from build123d import *

# Parameters (mm, degrees)
SKETCH_1_R               = 11
SKETCH_1_R_2             = 1.25
EXTRUDE_1_DEPTH          = 2
SKETCH_2_R               = 5
SKETCH_2_R_2             = 2.5
EXTRUDE_2_DEPTH          = 10
CUT_EXTRUDE_1_REACH      = 21.647
CUT_EXTRUDE_1_END_RADIUS = 5
SKETCH_3_R               = 1.5


with BuildPart() as part:
    # 草圖1 → 填料-伸長1 (new body)
    with BuildSketch(Plane(origin=(0, 0, 0), x_dir=(1, 0, 0), z_dir=(0, 1, 0))):
        with Locations(Location((0, 0, 0), (0, 0, 270))):
            Circle(SKETCH_1_R)
        with Locations(Location((0, 8, 0), (0, 0, 270))):
            Circle(SKETCH_1_R_2, mode=Mode.SUBTRACT)
        with Locations(Location((8, 0, 0), (0, 0, 270))):
            Circle(SKETCH_1_R_2, mode=Mode.SUBTRACT)
        with Locations(Location((0, -8, 0), (0, 0, 270))):
            Circle(SKETCH_1_R_2, mode=Mode.SUBTRACT)
        with Locations(Location((-8, 0, 0), (0, 0, 270))):
            Circle(SKETCH_1_R_2, mode=Mode.SUBTRACT)
    extrude(amount=EXTRUDE_1_DEPTH)

    # 草圖2 → 填料-伸長2 (add)
    with BuildSketch(Plane(origin=(0, 2, 0), x_dir=(1, 0, 0), z_dir=(0, 1, 0))):
        with Locations(Location((0, 0, 0), (0, 0, 270))):
            Circle(SKETCH_2_R)
        with Locations(Location((0, 0, 0), (0, 0, 270))):
            Circle(SKETCH_2_R_2, mode=Mode.SUBTRACT)
    extrude(amount=EXTRUDE_2_DEPTH)

    # 除料-伸長1: up to this cylinder (the profile starts inside it)
    cut_extrude_1_end = Plane(origin=(0, 9.5, 0), z_dir=(0, -1, 0)) * Cylinder(CUT_EXTRUDE_1_END_RADIUS, 54.294, mode=Mode.PRIVATE)
    # 草圖3 → 除料-伸長1 (cut, up to the surface)
    with BuildSketch(Plane.XY, mode=Mode.PRIVATE) as cut_extrude_1_sk1:
        with Locations(Location((0, 9.5, 0), (0, 0, 180))):
            Circle(SKETCH_3_R)
    cut_extrude_1_tool1 = extrude(cut_extrude_1_sk1.sketch, amount=CUT_EXTRUDE_1_REACH, mode=Mode.PRIVATE) & cut_extrude_1_end
    add(cut_extrude_1_tool1.solids().sort_by_distance((0, 9.5, 0))[0], mode=Mode.SUBTRACT)


solid = part.part
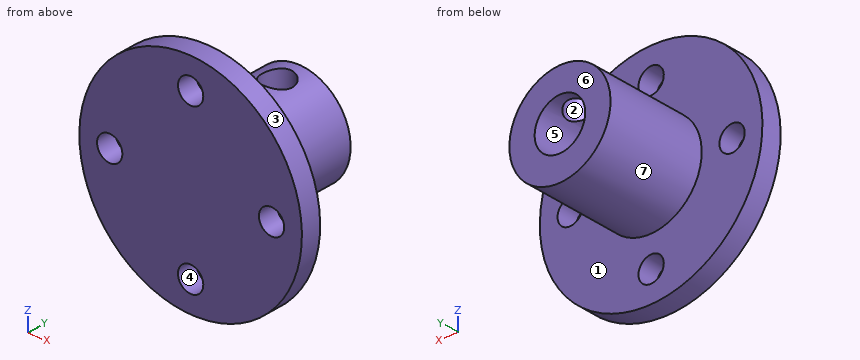
The model under review builds one solid part; all positions refer to its coordinate system, in mm. Face numbers are marked on the shaded views. A direction names the side the tool comes from. Give positions to 0.01 mm unless a question says otherwise; leave off trailing zeros. Order: outer loops, then holes, each group sorted by start corner. A loop starts at its lowest first (then second) coordinate and runs counter-clockwise, first axis right, second up. Notation, with made-up numbers: M 42,-5.75 L 54,-5.75 A35 ccw 54,31.25 Z; hole C 41.25,52.25 d6. An arc over 180 degrees is marked long. One line per question, with ' | ' between items. Start each with the question number.
1) Wall thickness on L1, parallel to X at y = 0.4, z = 0; L2, parallel to Y at x = 5.25, z = 7.25; L3, parallel to X at y = 10.5, z = -1.25: over which ranges is each line inside the solid? List them lowest first. Write a range as from..to.
2) Consider section B-B, the plane z = 0. Give the boundary of the cut face in (x, y).
3) Consider section C-C, the plane y = 1.5. Give the boundary of the cut face in (x, z).
4) Consider section A-A, the plane x = 0. Give the boundary of the cut face in (y, z).
5) For the marked faces 1, 2 and 3, list the 3-axis set-ups (+Z, -Z, +X, -X, +Y, -Y) from which the entire face can be reached by the end or side of a thin tool; tool diameter is ignored.
6) Clearance check with flat-ended pins moving along their axes: P1, Ø4, axis at y = 3.5, z = 7.5, coming from the -X side; P2, Ø4, axis at x = -8, y = 5.5, coming from the +Z side; P3, Ø8, axis at x = -7.5, z = 5, coming from the -Y side; P4, Ø3, axis at x = 0, z = 8, coming from the +Y side. State where each tip first meets the part, or that it passes through.
7) Mouldability with a two-part tool opening along Z and no side actions: class the marked faces 4, 5, 6 and 7 as pulls with the +Z half, pulls with the -Z half, needs draft (parallel to the pull), parting line crosses it, or undercut.
8) Consider section D-D, the plane x = -8. Give the boundary of the cut face in (y, z).
Found:
1) L1: x = -11..-9.25, -6.75..6.75, 9.25..11 | L2: y = 0..2 | L3: x = -4.84..-2.17, 2.17..4.84
2) outline: M -11,0 L -9.25,0 L -9.25,2 L -11,2 Z; M -6.75,0 L 6.75,0 L 6.75,2 L 5,2 L 5,12 L 2.5,12 L 2.5,2 L -2.5,2 L -2.5,12 L -5,12 L -5,2 L -6.75,2 Z; M 9.25,0 L 11,0 L 11,2 L 9.25,2 Z
3) outline: C 0,0 d22; hole C -8,0 d2.5; hole C 0,-8 d2.5; hole C 0,8 d2.5; hole C 8,0 d2.5
4) outline: M 0,-11 L 2,-11 L 2,-9.25 L 0,-9.25 Z; M 0,-6.75 L 2,-6.75 L 2,-5 L 12,-5 L 12,-2.5 L 2,-2.5 L 2,2.5 L 8,2.5 L 8,5 L 2,5 L 2,6.75 L 0,6.75 Z; M 0,9.25 L 2,9.25 L 2,11 L 0,11 Z; M 11,2.5 L 12,2.5 L 12,5 L 11,5 Z
5) face 1: +Y | face 2: +Z | face 3: +Y, -Y
6) P1: stops at x = -9.1 | P2: passes through | P3: stops at y = 0 | P4: stops at y = 2
7) face 4: undercut | face 5: undercut | face 6: needs draft | face 7: parting line crosses it
8) outline: M 0,-7.55 L 2,-7.55 L 2,-1.25 L 0,-1.25 Z; M 0,1.25 L 2,1.25 L 2,7.55 L 0,7.55 Z
